from build123d import *

# Parameters (mm, degrees)
SKETCH1_W               = 27
SKETCH1_H               = 20
SKETCH1_W_2             = 9
SKETCH1_H_2             = 3
BOSS_EXTRUDE1_DEPTH     = 3
BOSS_EXTRUDE2_START     = 3
SKETCH1_4_W             = 9
SKETCH1_4_H             = 3
BOSS_EXTRUDE2_DEPTH     = 4
SKETCH2_W               = 9
SKETCH2_H               = 6
BOSS_EXTRUDE3_DEPTH     = 3
BOSS_EXTRUDE4_START     = -4
SKETCH2_2_W             = 9
SKETCH2_2_H             = 6
BOSS_EXTRUDE4_DEPTH     = 2
SKETCH1_5_W             = 18
SKETCH1_5_H             = 3
BOSS_EXTRUDE5_DEPTH     = 10
SKETCH3_W               = 3
SKETCH3_H               = 26
BOSS_EXTRUDE6_DEPTH     = 7.54
SKETCH4_W               = 9
SKETCH4_H               = 3
BOSS_EXTRUDE7_DEPTH     = 7
SKETCH5_R               = 2.5
CUT_EXTRUDE1_DEPTH      = 4
CUT_EXTRUDE1_DEPTH_BACK = 24
SKETCH6_W               = 8
SKETCH6_H               = 8
SKETCH6_R               = 2.5
BOSS_EXTRUDE8_DEPTH     = 10


with BuildPart() as part:
    # Sketch1 → Boss-Extrude1 (new body)
    with BuildSketch(Plane(origin=(0, 0, 0), x_dir=(1, 0, 0), z_dir=(0, 1, 0))):
        Rectangle(SKETCH1_W, SKETCH1_H)
        with Locations((9, 11.5)):
            Rectangle(SKETCH1_W_2, SKETCH1_H_2)
        with Locations((9, -11.5)):
            Rectangle(SKETCH1_W_2, SKETCH1_H_2)
    extrude(amount=BOSS_EXTRUDE1_DEPTH)

    # Sketch1<4> → Boss-Extrude2 (add)
    with BuildSketch(Plane(origin=(0, 0, 0), x_dir=(1, 0, 0), z_dir=(0, 1, 0)).offset(BOSS_EXTRUDE2_START)):
        with Locations((9, -11.5)):
            Rectangle(SKETCH1_4_W, SKETCH1_4_H)
        with Locations((9, 11.5)):
            Rectangle(SKETCH1_4_W, SKETCH1_4_H)
    extrude(amount=BOSS_EXTRUDE2_DEPTH)

    # Sketch2 → Boss-Extrude3 (add)
    with BuildSketch(Plane(origin=(0, 7, 0), x_dir=(1, 0, 0), z_dir=(0, 1, 0))):
        with Locations((9, -10)):
            Rectangle(SKETCH2_W, SKETCH2_H)
        with Locations((9, 10)):
            Rectangle(SKETCH2_W, SKETCH2_H)
    extrude(amount=BOSS_EXTRUDE3_DEPTH)

    # Sketch2<2> → Boss-Extrude4 (add)
    with BuildSketch(Plane(origin=(0, 7, 0), x_dir=(1, 0, 0), z_dir=(0, 1, 0)).offset(BOSS_EXTRUDE4_START)):
        with Locations((9, -10)):
            Rectangle(SKETCH2_2_W, SKETCH2_2_H)
        with Locations((9, 10)):
            Rectangle(SKETCH2_2_W, SKETCH2_2_H)
    extrude(amount=BOSS_EXTRUDE4_DEPTH)

    # Sketch1<5> → Boss-Extrude5 (add)
    with BuildSketch(Plane(origin=(0, 0, 0), x_dir=(1, 0, 0), z_dir=(0, 1, 0))):
        Polygon((16.5, -13), (13.5, -13), (13.5, -10), (13.5, 10), (13.5, 13), (16.5, 13), align=None)
        with Locations((-4.5, -11.5)):
            Rectangle(SKETCH1_5_W, SKETCH1_5_H)
        with Locations((-4.5, 11.5)):
            Rectangle(SKETCH1_5_W, SKETCH1_5_H)
    extrude(amount=BOSS_EXTRUDE5_DEPTH)

    # Sketch3 → Boss-Extrude6 (add)
    with BuildSketch(Plane(origin=(0, 10, 0), x_dir=(1, 0, 0), z_dir=(0, 1, 0))):
        with Locations((15, 0)):
            Rectangle(SKETCH3_W, SKETCH3_H)
    extrude(amount=BOSS_EXTRUDE6_DEPTH)

    # Sketch4 → Boss-Extrude7 (add)
    with BuildSketch(Plane(origin=(0, 10, 0), x_dir=(1, 0, 0), z_dir=(0, 1, 0))):
        with Locations((9, 8.5)):
            Rectangle(SKETCH4_W, SKETCH4_H)
        with Locations((9, -8.5)):
            Rectangle(SKETCH4_W, SKETCH4_H)
    extrude(amount=BOSS_EXTRUDE7_DEPTH)

    # Sketch5 → Cut-Extrude1 (cut, two sides)
    with BuildSketch(Plane.XY.offset(10)) as cut_extrude1_sk:
        with Locations((9, 13.5)):
            Circle(SKETCH5_R)
    extrude(amount=CUT_EXTRUDE1_DEPTH, mode=Mode.SUBTRACT)
    extrude(cut_extrude1_sk.sketch, amount=-CUT_EXTRUDE1_DEPTH_BACK, mode=Mode.SUBTRACT)

    # Sketch6 → Boss-Extrude8 (add)
    with BuildSketch(Plane(origin=(16.5, 0, 0), x_dir=(0, 0, -1), z_dir=(1, 0, 0))):
        with Locations((17, 4)):
            Rectangle(SKETCH6_W, SKETCH6_H)
        with Locations((17, 4)):
            Circle(SKETCH6_R, mode=Mode.SUBTRACT)
    extrude(amount=-BOSS_EXTRUDE8_DEPTH)


solid = part.part
Can you work these out from the model? Positions are in its coordinate system, mm. A direction names the side the tool comes from. Coordinates: 2 decimals unless noted, no trailing zeros. Loops run counter-clockwise (first coordinate to the right, second up) from the corner with the lowest first, then second, coordinate; pieces in that order, holes last. Notation, with made-up numbers: (35, -1.75) - (56, -1.75) arc R15 cw to (56, 11.25) - close; hole circle Ø9 at (83.25, -2). An arc over 180 degrees is marked (long way). Put each result on its own line as item: value. Start each with the question number.
Item 1: Suppose I cut it at D-D (y = 4). Please give me the cut outline in (x, z).
Item 2: Suppose I cut it at A-A (x = 9). State how many separate pieces and enclosed holes the cut face has, and give its area (3 significant figures).
Item 3: Suppose I cut it at B-B (y = 13.5). Please give me the cut outline in (x, z), and give its area (3 significant figures).
Item 4: Which directions (+Z, -Z, +X, -X, +Y, -Y) give clear straight access to the entire face, cutting with the end or side of a thin tool? Please do faces 4 (the face through (0, 10, 11)), 5 (the face through (8.9, 10.8, -7)), 6 (the face through (12, 8, -17)), 7 (the face through (9, 5, -9)), 8 (the face through (6.5, 6, -15)).
Item 5: If I drill on line 1 along Z through (x, y) = (5.5, 5.5); line 2 along X through (y, z) = (12, 7.5); line 3 along Y through (x, z) = (9, -8.65), over which ranges is the centre line in solid material (lowest first)?
Item 6: For pin 1 (2.5 mm diameter, centred on x = 10, z = -8.5, fed in from -Y); pin 2 (16 mm diameter, centred on x = -0.5, z = 4, fed in from +Y); pin 3 (8 mm diameter, centred on x = -1.5, z = 3, fed in from +Y); pin 4 (4 mm diameter, centred on y = 6, z = -1, fed in from -X), each with a flat end and sliding along its axis, tell me the tip position at first contact or that it passes through.
Item 7: If we mould it in two halves opening along Z, with no side actions, what happens to faces 1 (the face through (12, 4, -21)), 2 (the face through (8.46, 11.06, -8.48)), 3 (the face through (13.5, 10, 0))? For each: +Z half, -Z half, draft (parallel to the pull), parting line (faces both ways), or undercut.
Item 8: Suppose I cut it at C-C (z = 9.5). Please give me the cut outline in (x, y).
Here are the results:
1. outline: (-13.5, -13) - (6.5, -13) - (6.5, -14.5) - (16.5, -14.5) - (16.5, 13) - (-13.5, 13) - (-13.5, 10) - (4.5, 10) - (4.5, 7) - (13.5, 7) - (13.5, -7) - (4.5, -7) - (4.5, -10) - (-13.5, -10) - close; (6.5, -21) - (16.5, -21) - (16.5, -19.5) - (6.5, -19.5) - close
2. separate pieces: 3
2. enclosed holes: 1
2. area: 206 mm²
3. outline: (4.5, -10) - (6.5, -10) - (6.5, -7) - (4.5, -7) - close; (4.5, 7) - (6.5, 7) - (6.5, 10) - (4.5, 10) - close; (11.5, -10) - (13.5, -10) - (13.5, -13) - (16.5, -13) - (16.5, 13) - (13.5, 13) - (13.5, 10) - (11.5, 10) - (11.5, 7) - (13.5, 7) - (13.5, -7) - (11.5, -7) - close
3. area: 102 mm²
4. face 4: +Z, -X, +Y
4. face 5: -X, +Y
4. face 6: -Z, +X, -X, +Y
4. face 7: -X
4. face 8: -Z, -X, +Y, -Y
5. line 1: -13 to -10, 10 to 13
5. line 2: 4.5 to 7, 11 to 16.5
5. line 3: 0 to 5, 7 to 11, 16 to 17
6. pin 1: y = 0
6. pin 2: y = 17
6. pin 3: y = 3
6. pin 4: x = 13.5
7. face 1: -Z half
7. face 2: draft
7. face 3: undercut
8. outline: (-13.5, 0) - (16.5, 0) - (16.5, 17.54) - (13.5, 17.54) - (13.5, 17) - (4.5, 17) - (4.5, 7) - (13.5, 7) - (13.5, 5) - (4.5, 5) - (4.5, 3) - (-13.5, 3) - close; hole circle Ø5 at (9, 13.5)
